```python
from build123d import *

# Parameters (mm, degrees)
BODY_SKETCH_W                                = 64
BODY_SKETCH_H                                = 25
BODY_DEPTH                                   = 160
BODY_ROD_HOLES_SKETCH_R                      = 5
BODY_ROD_HOLES_DEPTH                         = 10
BODY_PISTON_HOLES_SKETCH_R                   = 6.05
BODY_PISTON_HOLES_DEPTH                      = 91
TOP_SWITCH_GROOVES_DEPTH                     = 164.646723157
SHCS_MGT_HOLE_CHAM_SIZE                      = 0.3
SHCS_MGT_HOLE_PAT_COUNT                      = 2
SHCS_MGT_HOLE_PAT_PITCH                      = 60
SHCS_MGT_HOLE_CHAM_OF_SHCS_MGT_HOLE_PAT_SIZE = 0.3
SHCS_MGT_HOLE_BOT_TAP_AT_2_COUNT             = 2
SHCS_MGT_HOLE_BOT_TAP_AT_2_PITCH             = 60
ADJUSTER_NUT_DEPTH                           = 12
ADJUSTER_NUT_THREADS_SKETCH_W                = 1.8
ADJUSTER_NUT_THREADS_SKETCH_H                = 25
TAP_DRILL_FOR_M5X0_8_TAP1_D                  = 4.2
TAP_DRILL_FOR_M5X0_8_TAP1_DEPTH              = 4.5
TAP_DRILL_FOR_M5X0_8_TAP1_CSINK_D            = 5
TAP_DRILL_FOR_M5X0_8_TAP1_CSINK_ANGLE        = 90
TAP_DRILL_FOR_M5X0_8_TAP1_TIP                = 1.2618073
TAP_DRILL_FOR_M5X0_8_TAP2_D                  = 4.2
TAP_DRILL_FOR_M5X0_8_TAP2_DEPTH              = 4.5
TAP_DRILL_FOR_M5X0_8_TAP2_CSINK_D            = 5
TAP_DRILL_FOR_M5X0_8_TAP2_CSINK_ANGLE        = 90
TAP_DRILL_FOR_M5X0_8_TAP2_TIP                = 1.2618073
MOUNT_HOLES_1_D                              = 3.3
MOUNT_HOLES_1_DEPTH                          = 5.5
MOUNT_HOLES_1_CSINK_D                        = 4
MOUNT_HOLES_1_CSINK_ANGLE                    = 90
MOUNT_HOLES_1_TIP                            = 0.991420021
MOUNT_HOLES_2_D                              = 3.3
MOUNT_HOLES_2_DEPTH                          = 5.5
MOUNT_HOLES_2_CSINK_D                        = 4
MOUNT_HOLES_2_CSINK_ANGLE                    = 90
MOUNT_HOLES_2_TIP                            = 0.991420021
MOUNT_HOLES_3_D                              = 3.3
MOUNT_HOLES_3_DEPTH                          = 5.5
MOUNT_HOLES_3_CSINK_D                        = 4
MOUNT_HOLES_3_CSINK_ANGLE                    = 90
MOUNT_HOLES_3_TIP                            = 0.991420021
MOUNT_HOLES_4_D                              = 3.3
MOUNT_HOLES_4_DEPTH                          = 5.5
MOUNT_HOLES_4_CSINK_D                        = 4
MOUNT_HOLES_4_CSINK_ANGLE                    = 90
MOUNT_HOLES_4_TIP                            = 0.991420021


with BuildPart() as part:
    # Body_Sketch → Body (new body)
    with BuildSketch(Plane(origin=(0, 0, 0), x_dir=(0, 0, -1), z_dir=(1, 0, 0))):
        Rectangle(BODY_SKETCH_W, BODY_SKETCH_H)
    extrude(amount=BODY_DEPTH)

    # Body Rod Holes_Sketch → Body Rod Holes (cut)
    with BuildSketch(Plane.ZY):
        with Locations((-14, 0)):
            Circle(BODY_ROD_HOLES_SKETCH_R)
        with Locations(Location((14, 0, 0), (0, 0, 180))):
            Circle(BODY_ROD_HOLES_SKETCH_R)
    extrude(amount=-BODY_ROD_HOLES_DEPTH, mode=Mode.SUBTRACT)

    # Body Piston Holes_Sketch → Body Piston Holes (cut)
    with BuildSketch(Plane.ZY.offset(-10)):
        with Locations((14, 0)):
            Circle(BODY_PISTON_HOLES_SKETCH_R)
        with Locations((-14, 0)):
            Circle(BODY_PISTON_HOLES_SKETCH_R)
    extrude(amount=-BODY_PISTON_HOLES_DEPTH, mode=Mode.SUBTRACT)

    # Top Switch Grooves_Sketch → Top Switch Grooves (cut, through all)
    with BuildSketch(Plane.ZY):
        Polygon((23.35, 7.7), (29.65, 7.7), (29.65, 11.3), (29, 11.675277675), (29, 12.5), (24, 12.5), (24, 11.675277675), (23.35, 11.3), align=None)
        Polygon((-23.35, 11.3), (-23.35, 7.7), (-29.65, 7.7), (-29.65, 11.3), (-29, 11.675277675), (-29, 12.5), (-24, 12.5), (-24, 11.675277675), align=None)
    extrude(amount=-TOP_SWITCH_GROOVES_DEPTH, mode=Mode.SUBTRACT)

    # SHCS MGT Hole_Sketch → SHCS MGT Hole (revolve, cut)
    with BuildSketch(Plane.XY, mode=Mode.PRIVATE) as shcs_mgt_hole_sk:
        Polygon((30, 12.5), (25.25, 12.5), (25.25, 7.2), (27.25, 7.2), (27.25, -12.5), (30, -12.5), align=None)
    shcs_mgt_hole = revolve(shcs_mgt_hole_sk.sketch.rotate(Axis((30, -11.506886035, 0), (0, 1, 0)), 270), axis=Axis((30, -11.506886035, 0), (0, 1, 0)), mode=Mode.SUBTRACT)

    # SHCS MGT Hole Cham
    shcs_mgt_hole_cham_edges = [part.edges().sort_by_distance(p)[0] for p in [
        (30, 12.5, 4.75),
    ]]
    chamfer(shcs_mgt_hole_cham_edges, length=SHCS_MGT_HOLE_CHAM_SIZE)

    # SHCS MGT Hole Pat: SHCS MGT Hole ×2
    with Locations(*[(i * SHCS_MGT_HOLE_PAT_PITCH, 0, 0) for i in range(1, SHCS_MGT_HOLE_PAT_COUNT)]):
        add(shcs_mgt_hole, mode=Mode.SUBTRACT)

    # SHCS MGT Hole Cham of SHCS MGT Hole Pat
    shcs_mgt_hole_cham_of_shcs_mgt_hole_pat_edges = [part.edges().sort_by_distance(p)[0] for p in [
        (90, 12.5, 4.75),
    ]]
    chamfer(shcs_mgt_hole_cham_of_shcs_mgt_hole_pat_edges, length=SHCS_MGT_HOLE_CHAM_OF_SHCS_MGT_HOLE_PAT_SIZE)

    # SHCS MGT Hole Bot Tap Profile → SHCS MGT Hole Bot Tap (revolve, cut)
    with BuildSketch(Plane(origin=(30, -12.5, 0), x_dir=(0, 0, -1), z_dir=(1, 0, 0))):
        Polygon((0, 0), (0, 12.652366702), (2.75, 11), (2.75, 10), (3, 10), (3, 0.3), (3.3, 0), align=None)
    shcs_mgt_hole_bot_tap = revolve(axis=Axis((30, -18.85, 0), (0, 1, 0)), mode=Mode.SUBTRACT)

    # SHCS MGT Hole Bot Tap at 2: SHCS MGT Hole Bot Tap ×2
    with Locations(*[(i * SHCS_MGT_HOLE_BOT_TAP_AT_2_PITCH, 0, 0) for i in range(1, SHCS_MGT_HOLE_BOT_TAP_AT_2_COUNT)]):
        add(shcs_mgt_hole_bot_tap, mode=Mode.SUBTRACT)

    # Adjuster Nut_Sketch → Adjuster Nut (add)
    with BuildSketch(Plane.ZY):
        Polygon((-2.886751346, 11.5), (2.886751346, 11.5), (5.773502692, 6.5), (2.886751346, 1.5), (-2.886751346, 1.5), (-5.773502692, 6.5), align=None)
    extrude(amount=ADJUSTER_NUT_DEPTH)

    # Adjuster Nut Threads_Sketch → Adjuster Nut Threads (revolve, cut)
    with BuildSketch(Plane.XY, mode=Mode.PRIVATE) as adjuster_nut_threads_sk:
        with Locations((-5.9, 22)):
            Rectangle(ADJUSTER_NUT_THREADS_SKETCH_W, ADJUSTER_NUT_THREADS_SKETCH_H)
    revolve(adjuster_nut_threads_sk.sketch.rotate(Axis((-6.476, 6.5, 0), (1, 0, 0)), 270), axis=Axis((-6.476, 6.5, 0), (1, 0, 0)), mode=Mode.SUBTRACT)

    # Tap Drill for M5x0.8 Tap1
    with Locations(Plane.XY.offset(32)):
        with Locations((45, 0), (152, 0)):
            CounterSinkHole(TAP_DRILL_FOR_M5X0_8_TAP1_D / 2, TAP_DRILL_FOR_M5X0_8_TAP1_CSINK_D / 2, depth=TAP_DRILL_FOR_M5X0_8_TAP1_DEPTH, counter_sink_angle=TAP_DRILL_FOR_M5X0_8_TAP1_CSINK_ANGLE)
            with Locations((0, 0, -(TAP_DRILL_FOR_M5X0_8_TAP1_DEPTH + TAP_DRILL_FOR_M5X0_8_TAP1_TIP / 2))):  # 118° drill point
                Cone(0, TAP_DRILL_FOR_M5X0_8_TAP1_D / 2, TAP_DRILL_FOR_M5X0_8_TAP1_TIP, mode=Mode.SUBTRACT)

    # Tap Drill for M5x0.8 Tap2
    with Locations(Plane(origin=(0, 0, -32), x_dir=(-1, 0, 0), z_dir=(0, 0, -1))):
        with Locations((-152, 0), (-45, 0)):
            CounterSinkHole(TAP_DRILL_FOR_M5X0_8_TAP2_D / 2, TAP_DRILL_FOR_M5X0_8_TAP2_CSINK_D / 2, depth=TAP_DRILL_FOR_M5X0_8_TAP2_DEPTH, counter_sink_angle=TAP_DRILL_FOR_M5X0_8_TAP2_CSINK_ANGLE)
            with Locations((0, 0, -(TAP_DRILL_FOR_M5X0_8_TAP2_DEPTH + TAP_DRILL_FOR_M5X0_8_TAP2_TIP / 2))):  # 118° drill point
                Cone(0, TAP_DRILL_FOR_M5X0_8_TAP2_D / 2, TAP_DRILL_FOR_M5X0_8_TAP2_TIP, mode=Mode.SUBTRACT)

    # Mount_Holes_1
    with Locations(Plane.XY.offset(32)):
        with Locations((30, -4.75), (90, -4.75)):
            CounterSinkHole(MOUNT_HOLES_1_D / 2, MOUNT_HOLES_1_CSINK_D / 2, depth=MOUNT_HOLES_1_DEPTH, counter_sink_angle=MOUNT_HOLES_1_CSINK_ANGLE)
            with Locations((0, 0, -(MOUNT_HOLES_1_DEPTH + MOUNT_HOLES_1_TIP / 2))):  # 118° drill point
                Cone(0, MOUNT_HOLES_1_D / 2, MOUNT_HOLES_1_TIP, mode=Mode.SUBTRACT)

    # Mount_Holes_2
    with Locations(Plane(origin=(0, 0, -32), x_dir=(-1, 0, 0), z_dir=(0, 0, -1))):
        with Locations((-90, -4.75), (-30, -4.75)):
            CounterSinkHole(MOUNT_HOLES_2_D / 2, MOUNT_HOLES_2_CSINK_D / 2, depth=MOUNT_HOLES_2_DEPTH, counter_sink_angle=MOUNT_HOLES_2_CSINK_ANGLE)
            with Locations((0, 0, -(MOUNT_HOLES_2_DEPTH + MOUNT_HOLES_2_TIP / 2))):  # 118° drill point
                Cone(0, MOUNT_HOLES_2_D / 2, MOUNT_HOLES_2_TIP, mode=Mode.SUBTRACT)

    # Mount_Holes_3
    with Locations(Plane.XY.offset(32)):
        with Locations((30, 4.75), (90, 4.75)):
            CounterSinkHole(MOUNT_HOLES_3_D / 2, MOUNT_HOLES_3_CSINK_D / 2, depth=MOUNT_HOLES_3_DEPTH, counter_sink_angle=MOUNT_HOLES_3_CSINK_ANGLE)
            with Locations((0, 0, -(MOUNT_HOLES_3_DEPTH + MOUNT_HOLES_3_TIP / 2))):  # 118° drill point
                Cone(0, MOUNT_HOLES_3_D / 2, MOUNT_HOLES_3_TIP, mode=Mode.SUBTRACT)

    # Mount_Holes_4
    with Locations(Plane(origin=(0, 0, -32), x_dir=(-1, 0, 0), z_dir=(0, 0, -1))):
        with Locations((-90, 4.75), (-30, 4.75)):
            CounterSinkHole(MOUNT_HOLES_4_D / 2, MOUNT_HOLES_4_CSINK_D / 2, depth=MOUNT_HOLES_4_DEPTH, counter_sink_angle=MOUNT_HOLES_4_CSINK_ANGLE)
            with Locations((0, 0, -(MOUNT_HOLES_4_DEPTH + MOUNT_HOLES_4_TIP / 2))):  # 118° drill point
                Cone(0, MOUNT_HOLES_4_D / 2, MOUNT_HOLES_4_TIP, mode=Mode.SUBTRACT)


solid = part.part
```
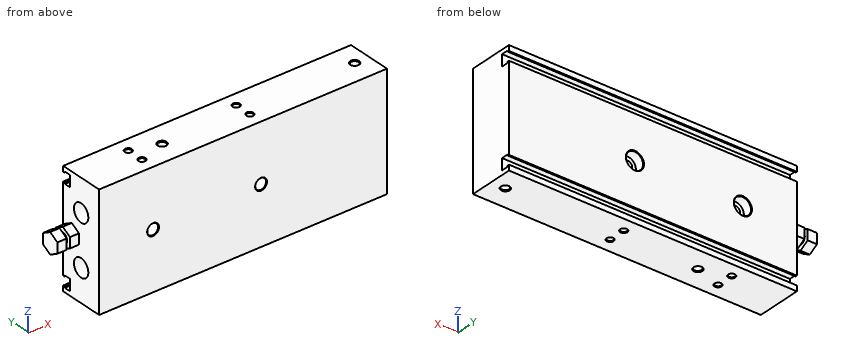
Geometry check sheet. Reference: the model listing, model coordinates, mm. Give positions to 0.01 mm unless a question says otherwise; leave off trailing zeros. Loops run counter-clockwise (first coordinate to the right, second up) from the corner with the lowest first, then second, coordinate; pieces in that order, holes last. Notation, with made-up numbers: M -31,62.25 L -26,62.25 A24 cw -26,72.25 Z; hole C 85,10 d10. An arc over 180 degrees is marked long. Answer as CSV lines item,"result".
Item 1: Cross-section at A-A on y = -9.5. Record the cut outline in (x, z).
Values:
outline,"M 0,-32 L 160,-32 L 160,32 L 0,32 Z; hole C 30,0 d6; hole C 90,0 d6"
Item 2: Material ranges on line 1 (X direction, y = 0, z = -29.85); line 2 (Z direction, x = 73.5, y = 7.75); line 3 (Y direction, x = 30, z = -29.25), recorded low to high.
Values:
line 1,"x = 0 to 42.9, 47.1 to 149.9, 154.1 to 160"
line 2,"z = -32 to -29.65, -23.35 to 23.35, 29.65 to 32"
line 3,"y = -12.5 to -6.4, -3.1 to 3.1, 6.4 to 7.7, 11.53 to 12.5"
Item 3: Depth check by flat-ended pin: P1, Ø4.5, axis at x = 30, z = 0, coming from the +Y side; P2, Ø9.5, axis at y = 1, z = -16, coming from the -X side; P3, Ø5, axis at x = 91.5, z = 0, coming from the +Y side; P4, Ø9, axis at y = 0, z = -14, coming from the -X side. Enter the tip coordinate at first touch or a pass-through.
Values:
P1,"passes through"
P2,"stops at x = 0"
P3,"stops at y = 7.2"
P4,"stops at x = 101"
Item 4: Cross-section at B-B on x = 145.5. Record the cut outline in (y, z), and give its area (3 significant figures).
Values:
outline,"M -12.5,-32 L 12.5,-32 L 12.5,-29 L 11.68,-29 L 11.3,-29.65 L 7.7,-29.65 L 7.7,-23.35 L 11.3,-23.35 L 11.68,-24 L 12.5,-24 L 12.5,24 L 11.68,24 L 11.3,23.35 L 7.7,23.35 L 7.7,29.65 L 11.3,29.65 L 11.68,29 L 12.5,29 L 12.5,32 L -12.5,32 Z"
area,"1,540 mm²"
Item 5: Cross-section at D-D on z = 0. Count the separate pieces of the cut face and the enclosed holes in it, and give its area (3 significant figures).
Values:
separate pieces,"3"
enclosed holes,"0"
area,"3,790 mm²"
Item 6: Cross-section at C-C on z = 14. Record the cut outline in (x, y).
Values:
outline,"M 0,-12.5 L 160,-12.5 L 160,12.5 L 0,12.5 L 0,5 L 10,5 L 10,6.05 L 101,6.05 L 101,-6.05 L 10,-6.05 L 10,-5 L 0,-5 Z"
